Autodesk Inventor part; units mm, degrees
ref_plane "Начальная плоскость" through (0, 0, 40) normal (0, 0, 1) x (1, 0, 0)
ref_plane "Конечная плоскость" through (0, 0, 360) normal (0, 0, 1) x (1, 0, 0)
ref_plane "РабПлоскость4" through (43.57, -400, 40) normal (0, 0, -1) x (-1, 0, 0)
ref_plane "Начальная плоскость" through (0, 0, 40) normal (0, 0, 1) x (1, 0, 0)
ref_plane "Конечная плоскость" through (0, 0, 360) normal (0, 0, 1) x (1, 0, 0)
sketch "Эскиз" plane through (0, 0, 0) normal (0, 0, 1) x (1, 0, 0)
  line L0 (-1.43, 0) -> (-1.43, 40)
  line L1 (-1.43, 40) -> (43.57, 40)
  line L2 (43.57, 40) -> (43.57, 38.1774)
  line L3 (39.9881, 34.1993) -> (11.2338, 31.1771)
  line L4 (4.07, 23.221) -> (4.07, 0)
  line L5 (4.07, 0) -> (-1.43, 0) construction
  line L6 (23.82, 40) -> (23.82, 32.5) construction
  line L7 (43.57, 34.5758) -> (43.57, 32.5) construction
  line L8 (43.57, 32.5) -> (23.82, 32.5) construction
  line L9 (0, 15) -> (0, -27) construction
  line L10 (-5.539, 0) -> (16.0067, 0) construction
  line L11 (-1.43, 0) -> (-1.43, -40)
  line L12 (-1.43, -40) -> (43.57, -40)
  line L13 (43.57, -40) -> (43.57, -38.1774)
  line L14 (39.9881, -34.1993) -> (11.2338, -31.1771)
  line L15 (4.07, -23.221) -> (4.07, 0)
  arc A0 (11.2338, 31.1771) -> (4.07, 23.221) centre (12.07, 23.221) ccw
  arc A1 (4.07, -23.221) -> (11.2338, -31.1771) centre (12.07, -23.221) ccw
  arc A2 (39.9881, 34.1993) -> (43.57, 38.1774) centre (39.57, 38.1774) ccw
  arc A3 (43.57, -38.1774) -> (39.9881, -34.1993) centre (39.57, -38.1774) ccw
  line L16 (0, 56) -> (0, -56) construction
  line L17 (-15.5135, 0) -> (54.308, 0) construction
  point P0 (4.07, 30.4242)
  point P1 (43.57, -34.5758)
  point P2 (4.07, -30.4242)
  point P3 (23.82, -40)
  point P4 (23.82, -32.5)
  dimension "d0" = 5.5
  dimension "d1" = 40
  dimension "d2" = 45
  dimension "d3" = 7.5
  dimension "d4" = 19.75
  dimension "d5" = 2.0758
  dimension "d23" = 8
  dimension "d24" = 4
  dimension "d25" = 1.43
extrude "Тело" add sketch "Эскиз" along normal up to surface (320 mm away) from surface at 40
sketch "Sketch3" plane through (0, 0, 0) normal (0, 0, 1) x (1, 0, 0)
  line L0 (0, 0) -> (10, 0)
ref_plane "Work Plane3" through (0, 0, 0) normal (0, -1, 0) x (1, 0, 0)
sketch "Sketch4" plane through (0, 0, 0) normal (0, -1, 0) x (1, 0, 0)
  line L0 (-2, 40) -> (12, 40)
  line L1 (-2, 360) -> (12, 360)
  dimension "d29" = 320
ref_plane "РабПлоскость4" through (43.57, -400, 40) normal (0, 0, -1) x (-1, 0, 0)
split "Разделение1" plane through (43.57, -400, 40) removes the side toward (0, 0, -1)
ref_plane "РабПлоскость5" through (43.57, 270, 360) normal (0, 0, 1) x (1, 0, 0)
split "Разделение2" plane through (43.57, 270, 360) removes the side toward (0, 0, 1)
equation "\"d0\" = G_T"
equation "\"d1\" = 0.5 * G_H"
equation "\"d2\" = G_W"
equation "\"d3\" = G_T1"
equation "\"d4\" = G_C"
equation "\"d23\" = G_IR"
equation "\"d24\" = G_ER"
equation "\"d25\" = ex"
equation "\"d6\" = G_L"
equation "\"G_W\" = 45"
equation "\"G_T\" = 5.5"
equation "\"G_T1\" = 7.5"
equation "\"G_NG\" = 0.105104"
equation "\"G_ER\" = 4"
equation "\"G_IR\" = 8"
equation "\"G_C\" = 19.75"
equation "\"G_L\" = d29"
equation "\"ex\" = 1.43"
properties part number "ISO 657/11 - CH 80 x 8 - 320" material "Сталь, мягкая"
Design review of the part built by this model. Coordinates are the model's own, in mm. A direction names the side the tool comes from. Coordinates: 2 decimals unless noted, no trailing zeros. Write each loop counter-clockwise with the first axis right and the second up, starting at its lowest first coordinate (ties: lowest second). Pieces come first, ordered by that corner, then holes.
1) Machinability: for faces 1 (the flat face through (25.81, 32.71, 197.76)), 2 (the flat face through (3, 0, 40)), which of the approach directions +Z, -Z, +X, -X, +Y, -Y give a long, thin tool a straight path to every point of the face, cutting with its end or side? Answer none if there is none.
2) Mouldability with a two-part tool opening along Y and no side actions: class faces 3 (the cylindrical face through (6.07, 28.51, 197.76)), 4 (the flat face through (21, 40, 198)), 5 (the flat face through (-1.43, -1, 198)) as +Y half, -Y half, draft (parallel to the pull), parting line (faces both ways), or undercut.
3) Add section B-B (x = 20). Write out the cut boundary in (y, z), plus the area to 3 significant figures.
4) Insertion check: pin 1 (23 mm diameter, centred on y = 0, z = 148, fed in from +X). The pin has a flat end and moves straight along its axis. Give the tip position at first contact, or say it passes through.
5) Add section A-A (z = 311.5). Write out the cut boundary in (x, y), plus the area to 3 significant figures.
6) Add section C-C (y = 19). Write out the cut boundary in (x, z), plus the area to 3 significant figures.
7) Add section D-D (x = 36). Write out the cut boundary in (y, z), plus the area to 3 significant figures.
8) To check wall thickness, follow L1, parallel to Y at x = 39.5, z = 71; L2, parallel to X at y = -1.5, z = 109; L3, parallel to Y at x = 14, z = 238. State the ranges of each line that lie inside material, in increasing order.
Check result:
1. face 1: +Z, -Z, +X
1. face 2: -Z, +X, -X, +Y, -Y
2. face 3: undercut
2. face 4: +Y half
2. face 5: draft
3. outline: (-40, 40) - (-32.1, 40) - (-32.1, 360) - (-40, 360) - close; (32.1, 40) - (40, 40) - (40, 360) - (32.1, 360) - close
3. area: 5,060 mm2
4. pin 1: stops at x = 4.07
5. outline: (-1.43, -40) - (43.57, -40) - (43.57, -38.18) arc R4 ccw to (39.99, -34.2) - (11.23, -31.18) arc R8 cw to (4.07, -23.22) - (4.07, 23.22) arc R8 cw to (11.23, 31.18) - (39.99, 34.2) arc R4 ccw to (43.57, 38.18) - (43.57, 40) - (-1.43, 40) - close
5. area: 1,050 mm2
6. outline: (-1.43, 40) - (4.07, 40) - (4.07, 360) - (-1.43, 360) - close
6. area: 1,760 mm2
7. outline: (-40, 40) - (-33.78, 40) - (-33.78, 360) - (-40, 360) - close; (33.78, 40) - (40, 40) - (40, 360) - (33.78, 360) - close
7. area: 3,980 mm2
8. L1: y = -40 to -34.15, 34.15 to 40
8. L2: x = -1.43 to 4.07
8. L3: y = -40 to -31.47, 31.47 to 40
